Geometry: final body of the model. Coordinates: model frame, mm. Coordinates: 2 decimals unless noted, no trailing zeros. Loops run counter-clockwise (first coordinate to the right, second up) from the corner with the lowest first, then second, coordinate; pieces in that order, holes last. Notation, with made-up numbers: (31, 82) - (43, 82) arc R20 ccw to (43, 96) - close; hole circle Ø3 at (46, 79). An arc over 180 degrees is marked (long way). Return JSON: item names as keys, results as strings.
from build123d import *

# Parameters (mm, degrees)
SKETCH_1_W      = 166
SKETCH_1_H      = 160
EXTRUDE_1_DEPTH = 2
MM_2_D          = 4
MM_2_DEPTH      = 10
MM_2_TIP        = 1.201721238


with BuildPart() as part:
    # 草图1 → 凸台-拉伸1 (new body)
    with BuildSketch(Plane(origin=(0, 0, 0), x_dir=(1, 0, 0), z_dir=(0, 1, 0))):
        Rectangle(SKETCH_1_W, SKETCH_1_H)
    extrude(amount=EXTRUDE_1_DEPTH)

    # 大小mm 暗销孔2
    with Locations(Plane(origin=(45.636831669, 2.8, 467.05931397), x_dir=(0.07852837759024327, 0, 0.9969118787099711), z_dir=(0, 1, 0))):
        with Locations((-404.949854974, -103.656881575), (-403.897574678, -90.298262111), (-432.80801916, -88.020939161), (-433.860299457, -101.379558625), (-547.50825363, -92.42732358), (-518.597809147, -94.70464653), (-517.545528888, -81.346027355), (-546.45597337, -79.068704405)):
            Hole(MM_2_D / 2, depth=MM_2_DEPTH)
            with Locations((0, 0, -(MM_2_DEPTH + MM_2_TIP / 2))):  # 118° drill point
                Cone(0, MM_2_D / 2, MM_2_TIP, mode=Mode.SUBTRACT)


solid = part.part
Item 1: Section query A-A, the plane z = 71.5. Return loops of the section in (x, y), and give its area (3 significant figures).
Worked out:
{"outline": "(-83, 0) - (-78.1, 0) - (-78.1, 2) - (-83, 2) - close; (-74.1, 0) - (83, 0) - (83, 2) - (-74.1, 2) - close", "area": "324 mm^2"}
Item 2: Mould query, pull axis Z, two halves, no side actions, for faces 1 (the face through (-1, 0, -1)), 2 (the face through (-74.103, 0.986, -71.396)). Classes: +Z half, -Z half, draft (parallel to the pull), parting line (faces both ways), or undercut.
Worked out:
{"face 1": "draft", "face 2": "undercut"}
Item 3: Ray query, probe 1 along Z at (x, y) = (-76.1, 0.7); probe 2 along X at (y, z) = (1.45, -42.5). Return the intervals inside material, ascending. Write a range as from..to.
Worked out:
{"probe 1": "-80..-73.5, -69.5..-44.5, -40.5..40.5, 44.5..69.5, 73.5..80", "probe 2": "-83..-78.1, -74.1..83"}
